Part model, mm, in its own coordinate system. Face numbers are marked on the shaded views. A direction names the side the tool comes from. Round coordinates to 2 decimals unless told otherwise and drop trailing zeros. Write each loop counter-clockwise with the first axis right and the second up, starting at its lowest first coordinate (ties: lowest second). Pieces come first, ordered by that corner, then holes.
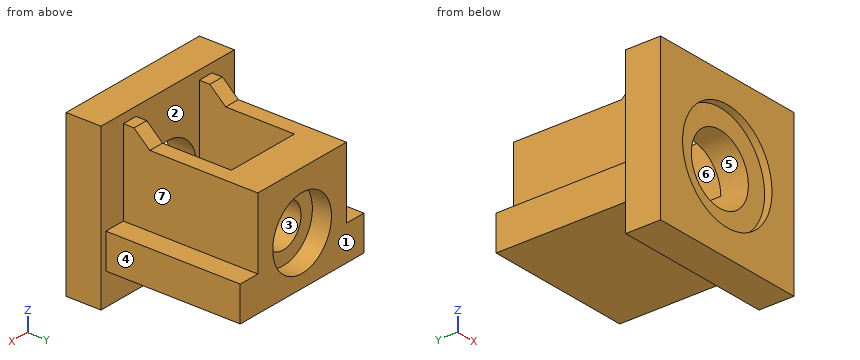
```python
from build123d import *

# Parameters (mm, degrees)
F0_W      = 152
F0_H      = 152
F1_DEPTH  = 33
F3_DEPTH  = 127
F4_R      = 20.5
F5_DEPTH  = 156
F4_R_2    = 32.5
F6_DEPTH  = 119
F4_R_3    = 51
F7_DEPTH  = 7
F8_R      = 33.5
F9_DEPTH  = 18
F10_W     = 72
F10_H     = 90
F11_DEPTH = 54
F13_DEPTH = 14.5
F15_DEPTH = 14.5


with BuildPart() as f1:
    # F0 (on Front) → F1 (new body)
    with BuildSketch(Plane.XZ):
        Rectangle(F0_W, F0_H)
    extrude(amount=-F1_DEPTH)

    # F2 (on face) → F3 (join)
    with BuildSketch(Plane(origin=(0, 33, 0), x_dir=(-1, 0, 0), z_dir=(0, 1, 0))):
        Polygon((50.5, 54), (-50.5, 54), (-50.5, -13), (-70.5, -13), (-70.5, -46), (70.5, -46), (70.5, -13), (50.5, -13), align=None)
    extrude(amount=F3_DEPTH)

    # F4 (on Front) → F5 (cut)
    with BuildSketch(Plane.XZ):
        Circle(F4_R)
    extrude(amount=-F5_DEPTH, mode=Mode.SUBTRACT)

    # F4 (on Front) → F6 (cut)
    with BuildSketch(Plane.XZ):
        Circle(F4_R_2)
        Circle(F4_R, mode=Mode.SUBTRACT)
        Circle(F4_R)
    extrude(amount=-F6_DEPTH, mode=Mode.SUBTRACT)

    # F4 (on Front) → F7 (cut)
    with BuildSketch(Plane.XZ):
        Circle(F4_R_3)
        Circle(F4_R_2, mode=Mode.SUBTRACT)
    extrude(amount=-F7_DEPTH, mode=Mode.SUBTRACT)

    # F8 (on face) → F9 (cut)
    with BuildSketch(Plane(origin=(0, 160, 0), x_dir=(-1, 0, 0), z_dir=(0, 1, 0))):
        Circle(F8_R)
    extrude(amount=-F9_DEPTH, mode=Mode.SUBTRACT)

    # F10 (on face) → F11 (cut)
    with BuildSketch(Plane.XY.offset(54)):
        with Locations((0, 78)):
            Rectangle(F10_W, F10_H)
    extrude(amount=-F11_DEPTH, mode=Mode.SUBTRACT)

    # F12 (on face) → F13 (join)
    with BuildSketch(Plane.YZ.offset(50.5)):
        Polygon((33, 67.5), (33, 54), (58, 54), (43, 67.5), align=None)
    extrude(amount=-F13_DEPTH)

    # F14 (on face) → F15 (join)
    with BuildSketch(Plane(origin=(-50.5, 0, 0), x_dir=(0, -1, 0), z_dir=(-1, 0, 0))):
        Polygon((-58, 54), (-33, 54), (-33, 67.5), (-43, 67.5), align=None)
    extrude(amount=-F15_DEPTH)


solid = f1.part
```
Q1. Cut at B-B on z = -4. Write the cut outline in (x, y), plus the area to 3 significant figures.
Values follow:
outline: (-76, 0) - (-50.84, 0) - (-50.84, 7) - (-32.25, 7) - (-32.25, 119) - (-20.11, 119) - (-20.11, 142) - (-33.26, 142) - (-33.26, 160) - (-50.5, 160) - (-50.5, 33) - (-76, 33) - close; (20.11, 119) - (32.25, 119) - (32.25, 7) - (50.84, 7) - (50.84, 0) - (76, 0) - (76, 33) - (50.5, 33) - (50.5, 160) - (33.26, 160) - (33.26, 142) - (20.11, 142) - close
area: 7,780 mm2
Q2. Cut at C-C on y = 93. Write the cut outline in (x, z), plus the area to 3 significant figures.
Values follow:
outline: (-70.5, -46) - (70.5, -46) - (70.5, -13) - (50.5, -13) - (50.5, 54) - (36, 54) - (36, 0) - (32.5, 0) arc R32.5 cw to (-32.5, 0) - (-36, 0) - (-36, 54) - (-50.5, 54) - (-50.5, -13) - (-70.5, -13) - close
area: 5,870 mm2
Q3. Drop flat-ended pins along their axis: pin 1 (8 mm diameter, centred on x = 24, y = 53.5, fed in from +Z); pin 2 (24 mm diameter, centred on y = 97.5, z = 34.5, fed in from -X); pin 3 (22 mm diameter, centred on x = 63.5, y = 113, fed in from +Z). Give the stop position or say it passes through.
Values follow:
pin 1: stops at z = -16.5
pin 2: stops at x = -50.5
pin 3: stops at z = -13
Q4. Which spindle directions (+Z, -Z, +X, -X, +Y, -Y) get a long thin tool onto all of the face, cutting with end or side? Do the marked faces 4, 5, 6 and 7. Say none if no direction does.
Values follow:
face 4: +Z, -Z, +X, +Y
face 5: -Y
face 6: +Z
face 7: +Z, +X, +Y
Q5. Cut at A-A on x = 0. Write the cut outline in (y, z), plus the area to 3 significant figures.
Values follow:
outline: (0, -76) - (33, -76) - (33, -46) - (160, -46) - (160, -33.5) - (142, -33.5) - (142, -20.5) - (119, -20.5) - (119, -32.5) - (7, -32.5) - (7, -51) - (0, -51) - close; (0, 51) - (7, 51) - (7, 32.5) - (33, 32.5) - (33, 76) - (0, 76) - close; (123, 20.5) - (142, 20.5) - (142, 33.5) - (160, 33.5) - (160, 54) - (123, 54) - close
area: 5,590 mm2
Q6. Wall check: L1, parallel to Z at x = 0, y = 156; L2, parallel to Z at x = 0, y = 130; L3, parallel to Y at x = -28.5, z = 17. Give the ranges that are in metal, low to high.
Values follow:
L1: z = -46 to -33.5, 33.5 to 54
L2: z = -46 to -20.5, 20.5 to 54
L3: y = 7 to 33, 123 to 142
Q7. Mould opens along Y. For the marked faces 1, 2 and 3 say: +Y half, -Y half, draft (parallel to the pull), parting line (faces both ways), or undercut.
Values follow:
face 1: +Y half
face 2: undercut
face 3: draft
Q8. Cut at D-D on x = 26.5. Write the cut outline in (y, z), plus the area to 3 significant figures.
Values follow:
outline: (0, -76) - (33, -76) - (33, -46) - (160, -46) - (160, -20.49) - (142, -20.49) - (142, 20.49) - (160, 20.49) - (160, 54) - (123, 54) - (123, 0) - (119, 0) - (119, -18.81) - (7, -18.81) - (7, -43.57) - (0, -43.57) - close; (0, 43.57) - (7, 43.57) - (7, 18.81) - (33, 18.81) - (33, 76) - (0, 76) - close
area: 8,910 mm2
